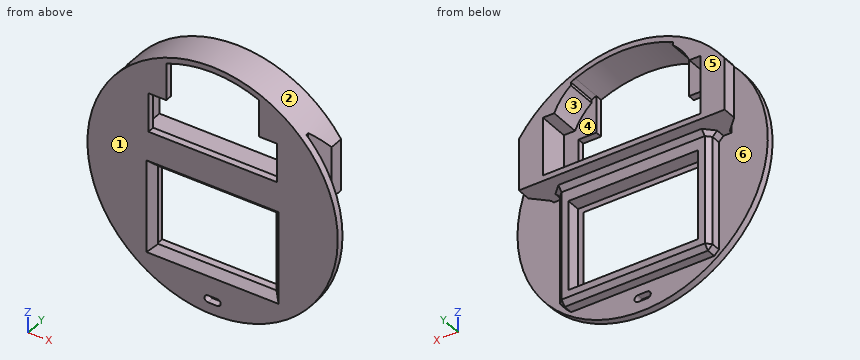
from build123d import *

# Parameters (mm, degrees)
SKETCH1_R                      = 27
SKETCH1_W                      = 25.5
SKETCH1_H                      = 17
BOSS_EXTRUDE1_DEPTH            = 1.5
BOSS_EXTRUDE2_START            = 6.6
BOSS_EXTRUDE2_DEPTH            = 6.6
CUT_EXTRUDE1_REACH             = 44.685
CUT_EXTRUDE1_END_RADIUS        = 27
CUT_EXTRUDE1_DIRECTION_2_DEPTH = 1.2
SKETCH1_5_W                    = 32.9
SKETCH1_5_H                    = 25.4
SKETCH1_5_W_2                  = 27.9
SKETCH1_5_H_2                  = 19.4
BOSS_EXTRUDE3_DEPTH            = 3
CHAMFER1_SIZE                  = 1.5
CHAMFER2_SIZE                  = 1


with BuildPart() as part:
    # Sketch1 → Boss-Extrude1 (new body)
    with BuildSketch(Plane(origin=(0, 0, 0), x_dir=(1, 0, 0), z_dir=(0, 1, 0))):
        with Locations(Location((0, 11.695639977, 0), (0, 0, 270))):
            Circle(SKETCH1_R)
        with BuildLine():
            Line((10, -4.1), (10, -12.087547362))
            ThreePointArc((10, -12.087547362), (0, -14.104360023), (-10, -12.087547362))
            Line((-10, -12.087547362), (-10, -4.1))
            Line((-10, -4.1), (-13.837653888, -4.1))
            Line((-13.837653888, -4.1), (-13.837653888, 4.3))
            Line((-13.837653888, 4.3), (13.837653888, 4.3))
            Line((13.837653888, 4.3), (13.837653888, -4.1))
            Line((13.837653888, -4.1), (10, -4.1))
        make_face(mode=Mode.SUBTRACT)
        with BuildLine():
            ThreePointArc((-1, 34.9), (-1.75, 35.65), (-1, 36.4))
            Line((-1, 36.4), (1, 36.4))
            ThreePointArc((1, 36.4), (1.75, 35.65), (1, 34.9))
            Line((1, 34.9), (-1, 34.9))
        make_face(mode=Mode.SUBTRACT)
        with Locations((0, 20.7)):
            Rectangle(SKETCH1_W, SKETCH1_H, mode=Mode.SUBTRACT)
    extrude(amount=-BOSS_EXTRUDE1_DEPTH)

    # Sketch1<3> → Boss-Extrude2 (add)
    with BuildSketch(Plane(origin=(0, 0, 0), x_dir=(1, 0, 0), z_dir=(0, 1, 0)).offset(BOSS_EXTRUDE2_START)):
        with BuildLine():
            Line((-16.45, 7.5), (-22.2, 7.5))
            Line((-22.2, 7.5), (-22.2, -3.671858193))
            ThreePointArc((-22.2, -3.671858193), (0, -15.304360023), (22.2, -3.671858193))
            Line((22.2, -3.671858193), (22.2, 7.5))
            Line((22.2, 7.5), (16.45, 7.5))
            Line((16.45, 7.5), (-16.45, 7.5))
        make_face()
        with BuildLine():
            Line((-17, -6.3), (-17, 6.3))
            Line((-17, 6.3), (17, 6.3))
            Line((17, 6.3), (17, -6.3))
            Line((17, -6.3), (14.582906959, -6.3))
            ThreePointArc((14.582906959, -6.3), (13.072174848, -8.850843183), (11, -10.971032764))
            Line((11, -10.971032764), (11, -11.641883456))
            ThreePointArc((11, -11.641883456), (10.502364214, -11.870020335), (10, -12.087547362))
            ThreePointArc((10, -12.087547362), (0, -14.104360023), (-10, -12.087547362))
            ThreePointArc((-10, -12.087547362), (-10.502364214, -11.870020335), (-11, -11.641883456))
            Line((-11, -11.641883456), (-11, -10.971032764))
            ThreePointArc((-11, -10.971032764), (-13.072174848, -8.850843183), (-14.582906959, -6.3))
            Line((-14.582906959, -6.3), (-17, -6.3))
        make_face(mode=Mode.SUBTRACT)
    extrude(amount=-BOSS_EXTRUDE2_DEPTH)

    # Cut-Extrude1: up to this cylinder (the profile starts inside it)
    cut_extrude1_end = Plane(origin=(0, 1.228571, -11.695639977), z_dir=(0, 1, 0)) * Cylinder(CUT_EXTRUDE1_END_RADIUS, 144.37, mode=Mode.PRIVATE)
    # Sketch2 → Cut-Extrude1 (cut, up to the surface)
    with BuildSketch(Plane.XY.offset(-6.3), mode=Mode.PRIVATE) as cut_extrude1_sk1:
        Polygon((-22.2, 3.6), (-19.2, 0.6), (-19.2, 0), (-22.2, 0), align=None)
    cut_extrude1_tool1 = extrude(cut_extrude1_sk1.sketch, amount=CUT_EXTRUDE1_REACH, mode=Mode.PRIVATE) & cut_extrude1_end
    add(cut_extrude1_tool1.solids().sort_by_distance((-21.057143, 1.228571, -6.3))[0], mode=Mode.SUBTRACT)
    # Sketch2 → Cut-Extrude1 (cut, up to the surface)
    with BuildSketch(Plane.XY.offset(-6.3), mode=Mode.PRIVATE) as cut_extrude1_sk2:
        Polygon((19.2, 0.6), (19.2, 0), (22.2, 0), (22.2, 3.6), align=None)
    cut_extrude1_tool2 = extrude(cut_extrude1_sk2.sketch, amount=CUT_EXTRUDE1_REACH, mode=Mode.PRIVATE) & cut_extrude1_end
    add(cut_extrude1_tool2.solids().sort_by_distance((21.057143, 1.228571, -6.3))[0], mode=Mode.SUBTRACT)

    # Sketch2 → Cut-Extrude1 direction 2 (cut)
    with BuildSketch(Plane.XY.offset(-6.3)):
        Polygon((-22.2, 3.6), (-19.2, 0.6), (-19.2, 0), (-22.2, 0), align=None)
        Polygon((19.2, 0.6), (19.2, 0), (22.2, 0), (22.2, 3.6), align=None)
    extrude(amount=-CUT_EXTRUDE1_DIRECTION_2_DEPTH, mode=Mode.SUBTRACT)

    # Sketch1<5> → Boss-Extrude3 (add)
    with BuildSketch(Plane(origin=(0, 0, 0), x_dir=(1, 0, 0), z_dir=(0, 1, 0))):
        with Locations((0, 20.2)):
            Rectangle(SKETCH1_5_W, SKETCH1_5_H)
        with Locations((0, 20.7)):
            Rectangle(SKETCH1_5_W_2, SKETCH1_5_H_2, mode=Mode.SUBTRACT)
    extrude(amount=BOSS_EXTRUDE3_DEPTH)

    # Chamfer1
    chamfer1_edges = [part.edges().sort_by_distance(p)[0] for p in [
        (-12.75, -1.5, -20.7),
        (0, -1.5, -12.2),
        (0, -1.5, -29.2),
        (12.75, -1.5, -20.7),
    ]]
    chamfer(chamfer1_edges, length=CHAMFER1_SIZE - 0.0001)  # a hair under: the kernel refuses the full size

    # Chamfer2
    chamfer2_edges = [part.edges().sort_by_distance(p)[0] for p in [
        (16.45, 3, -20.2),
        (16.45, 1.5, -7.5),
        (0, 3, -32.9),
        (16.45, 1.5, -32.9),
        (-16.45, 1.5, -32.9),
        (-16.45, 1.5, -7.5),
        (-16.45, 3, -20.2),
        (0, 3, -7.5),
    ]]
    chamfer(chamfer2_edges, length=CHAMFER2_SIZE)


solid = part.part
The listing builds one solid part. Answer for the finished solid, in the listing's coordinates (mm). Face numbers are marked on the shaded views. A direction names the side the tool comes from. Give positions to 0.01 mm unless a question says otherwise; leave off trailing zeros. Write each loop counter-clockwise with the first axis right and the second up, starting at its lowest first coordinate (ties: lowest second). Pieces come first, ordered by that corner, then holes. Notation, with made-up numbers: (69, 28.25) - (92, 28.25) arc R12 cw to (92, 33.25) - close; hole circle Ø9 at (52, 49). An arc over 180 degrees is marked (long way). One line per question, with ' | ' between items. Start each with the question number.
1. Section B-B, the plane z = -35.65 is taken. Determine the outline of the cut face in (x, y).
2. Straight lines are drawn through the part: line 1 (Z direction, x = 0.5, y = 1.75); line 2 (X direction, y = 1.5, z = -15.5); line 3 (Z direction, x = -8, y = 1.5). For each, find the intervals that lie inside material, in ascending order.
3. Given P1, Ø3.5, axis at y = 5.5, z = 0, coming from the +X side; P2, Ø2.5, axis at x = 5.5, y = 2, coming from the +Z side; P3, Ø1.5, axis at y = 5, z = -27, coming from the -X side; P4, Ø4, axis at y = 2, z = 6.5, coming from the -X side, each flat-ended and moving along its own axis, determine where each tip first touches the part or whether it passes through.
4. Section A-A, the plane x = 0 is taken. Count the separate pieces of the cut face and the enclosed holes in it, then the cut area to 3 significant figures.
5. For the marked faces 4, 5 and 6, determine the directions among +Z, -Z, +X, -X, +Y, -Y from which every point of the face is accessible in a straight line to the end or side of a thin tool.
6. Determine the mould class of the marked faces 1, 2 and 3 for opening direction X: +X half, -X half, draft (parallel to the pull), parting line (faces both ways), or undercut.
Result:
1) outline: (-12.46, -1.5) - (-1.75, -1.5) - (-1.75, 0) - (-12.46, 0) - close; (1.75, -1.5) - (12.46, -1.5) - (12.46, 0) - (1.75, 0) - close
2) line 1: z = -32.9 to -30.4, -11 to -6.3, 14.1 to 15.3 | line 2: x = -16.45 to -13.95, 13.95 to 16.45 | line 3: z = -32.9 to -30.4, -11 to -6.3, 12.83 to 14.09
3) P1: stops at x = 22.2 | P2: stops at z = 14.97 | P3: passes through | P4: stops at x = -21.46
4) separate pieces: 4 | enclosed holes: 0 | area: 57.2 mm2
5) face 4: +Y | face 5: +Z, -Z, +X, -X, +Y | face 6: -Z
6) face 1: draft | face 2: parting line | face 3: undercut
